Verification items for the finished model (mm, model axes). A direction names the side the tool comes from. Round coordinates to 2 decimals unless told otherwise and drop trailing zeros. Use one line per item in the form item = value. Start each with the question number.
Item 1: Go/stop test with flat-tipped pins: pin 1 Ø3 at (x, z) = (5.5, 6) entering from -Y; pin 2 Ø1.5 at (y, z) = (-1.5, 4.5) entering from -X; pin 3 Ø7 at (x, y) = (0, 0) entering from +Z; pin 4 Ø2.5 at (x, y) = (0, 0) entering from +Z. Record where each tip stops, or that it passes through.
Item 2: Tool access check on faces 5 (the cylindrical face through (23.082, 8.325, 6.205)), 6 (the cylindrical face through (-0.86, -3.874, 7.638)), 7 (the cylindrical face through (-0.306, -1.378, 4.418)). Record the directions out of +Z, -Z, +X, -X, +Y, -Y that give a thin tool (end or side, any length) a straight path to the whole face; none if there is none.
Item 3: Release check for a two-part mould opening along Y. For faces 1 (the flat face through (9, 3, 2.54)), 2 (the flat face through (2, 0, 6.35)), 3 (the cylindrical face through (24.05, 13.33, 3.48)), 4 (the cylindrical face through (22.952, 12.204, 3.479)) record: +Y half, -Y half, draft (parallel to the pull), parting line (faces both ways), or undercut.
Item 4: Thickness scan on probe 1 along Y at (x, z) = (0, 4.3); probe 2 along Y at (x, z) = (-1.5, 6.5); probe 3 along X at (y, z) = (1.25, 4.25). Record the ranges inside material, lowest first. Write a range as [from, to].
from build123d import *

# Parameters (mm, degrees)
SKETCH1_R           = 1.411527177
SKETCH1_R_2         = 1.243983369
BOSS_EXTRUDE1_DEPTH = 8.89
SKETCH2_R           = 2.645579886
CUT_EXTRUDE1_DEPTH  = 4.445
FILLET1_R           = 3.556
SKETCH3_W           = 44.674996293
SKETCH3_H           = 31.668439698
CUT_EXTRUDE2_DEPTH  = 2.54
SKETCH4_R           = 3.96875
CUT_EXTRUDE3_DEPTH  = 2.54
CUT_EXTRUDE7_DEPTH  = 4.445


with BuildPart() as part:
    # Sketch1 → Boss-Extrude1 (new body)
    with BuildSketch(Plane.XY):
        with BuildLine():
            add(Edge.make_bspline(
                [(21.205268726, 12.646161991), (14.255823247, 10.148268513), (7.187400407, 8.811547849), (0, 8.636)],
                knots=[0.085210597, 0.085210597, 0.085210597, 0.085210597, 0.879863224, 0.879863224, 0.879863224, 0.879863224], degree=3))
            add(Edge.make_bspline(
                [(0, 8.636), (-0.12439204, 8.632961801), (-0.248819718, 8.630271408), (-0.373283033, 8.627928823)],
                knots=[0.879863224, 0.879863224, 0.879863224, 0.879863224, 0.893616244, 0.893616244, 0.893616244, 0.893616244], degree=3))
            ThreePointArc((-0.373283033, 8.627928823), (-8.155941991, -2.839208736), (5.065163845, -6.994613014))
            add(Edge.make_bspline(
                [(5.065163845, -6.994613014), (17.65304868, -2.514917498), (24.488656608, 3.25999298), (25.571987628, 10.33011842)],
                knots=[0.06260201, 0.06260201, 0.06260201, 0.06260201, 0.556375894, 0.556375894, 0.556375894, 0.556375894], degree=3))
            add(Edge.make_bspline(
                [(25.571987628, 10.33011842), (25.604508953, 10.542361808), (25.63184641, 10.755772424), (25.654, 10.97035027)],
                knots=[0.556375894, 0.556375894, 0.556375894, 0.556375894, 0.571198862, 0.571198862, 0.571198862, 0.571198862], degree=3))
            ThreePointArc((25.654, 10.97035027), (24.009383316, 13.347299726), (21.205268726, 12.646161991))
        make_face()
        Circle(SKETCH1_R, mode=Mode.SUBTRACT)
        with Locations((23.114, 10.97035027)):
            Circle(SKETCH1_R_2, mode=Mode.SUBTRACT)
    extrude(amount=BOSS_EXTRUDE1_DEPTH)

    # Sketch2 → Cut-Extrude1 (cut)
    with BuildSketch(Plane.XY.offset(8.89)):
        with Locations((23.114, 10.97035027)):
            Circle(SKETCH2_R)
    extrude(amount=-CUT_EXTRUDE1_DEPTH, mode=Mode.SUBTRACT)

    # Fillet1
    fillet1_edges = [part.edges().sort_by_distance(p)[0] for p in [
        (10.663514179, 9.764845798, 8.89),
        (-8.155941991, -2.839208736, 8.89),
        (17.427402091, -0.984924283, 8.89),
    ]]
    fillet(fillet1_edges, radius=FILLET1_R)

    # Sketch3 → Cut-Extrude2 (cut)
    with BuildSketch(Plane(origin=(0, 0, 0), x_dir=(-1, 0, 0), z_dir=(0, 0, -1))):
        with Locations((-8.365824592, 1.646921095)):
            Rectangle(SKETCH3_W, SKETCH3_H)
    extrude(amount=-CUT_EXTRUDE2_DEPTH, mode=Mode.SUBTRACT)

    # Sketch4 → Cut-Extrude3 (cut)
    with BuildSketch(Plane.XY.offset(8.89)):
        Circle(SKETCH4_R)
    extrude(amount=-CUT_EXTRUDE3_DEPTH, mode=Mode.SUBTRACT)

    # Sketch9 → Cut-Extrude7 (cut)
    with BuildSketch(Plane.XY.offset(8.89)):
        Polygon((21.408086702, 8.948234361), (14.616524105, 10.508926006), (20.791087942, 14.493017593), (23.324721169, 10.827396362), align=None)
    extrude(amount=-CUT_EXTRUDE7_DEPTH, mode=Mode.SUBTRACT)


solid = part.part
Output values:
q1.pin_1 = -7.62
q1.pin_2 = -8.6
q1.pin_3 = 6.35
q1.pin_4 = through
q2.face_5 = +Z, +Y
q2.face_6 = +Z
q2.face_7 = +Z, -Z
q3.face_1 = draft
q3.face_2 = undercut
q3.face_3 = +Y half
q3.face_4 = undercut
q4.probe_1 = [-8.64, -1.41], [1.41, 8.64]
q4.probe_2 = [-8.31, -3.67], [3.67, 8.31]
q4.probe_3 = [-8.55, -0.66], [0.66, 20.27]
